Source: CAD feature listing. Evaluate the final solid. Frame: model axes, mm. Round coordinates to 2 decimals unless told otherwise and drop trailing zeros. Write each loop counter-clockwise with the first axis right and the second up, starting at its lowest first coordinate (ties: lowest second). Pieces come first, ordered by that corner, then holes.
from build123d import *

# Parameters (mm, degrees)
SKETCH1_R                = 3.175
BOSS_EXTRUDE1_DEPTH      = 69.85
BOSS_EXTRUDE1_DEPTH_BACK = 69.85


with BuildPart() as part:
    # Sketch1 → Boss-Extrude1 (new body, two sides)
    with BuildSketch(Plane.XY) as boss_extrude1_sk:
        Polygon((6.284319593, 3.777652789), (-0.129383485, 7.331206807), (-6.413703078, 3.553554018), (-6.284319593, -3.777652789), (0.129383485, -7.331206807), (6.413703078, -3.553554018), align=None)
        Circle(SKETCH1_R, mode=Mode.SUBTRACT)
    extrude(amount=BOSS_EXTRUDE1_DEPTH)
    extrude(boss_extrude1_sk.sketch, amount=-BOSS_EXTRUDE1_DEPTH_BACK)


solid = part.part
1) Section query B-B on y = 0. Return the cut outline in (x, z) (3 decimals), then the cut area to 3 significant figures.
Taken from the geometry:
outline: (-6.351, -69.85) - (-3.175, -69.85) - (-3.175, 69.85) - (-6.351, 69.85) - close; (3.175, -69.85) - (6.351, -69.85) - (6.351, 69.85) - (3.175, 69.85) - close
area: 887 mm2
2) Section query C-C on x = -4.5. Return the cut outline in (y, z), then the cut area to 3 significant figures.
Taken from the geometry:
outline: (-4.77, -69.85) - (4.7, -69.85) - (4.7, 69.85) - (-4.77, 69.85) - close
area: 1,320 mm2
3) Pull-direction query (Y, two-part tool) for faces 1 (the face through (3.228, -5.469, 0.978)), 2 (the face through (-3.228, 5.469, 0.978)), 3 (the face through (-3, -2, -69.85)), 4 (the face through (-0.69, -3.1, -0.98)); classes: released by +Y, released by -Y, zero draft, split by the parting line, or undercut.
Taken from the geometry:
face 1: released by -Y
face 2: released by +Y
face 3: zero draft
face 4: undercut
4) Section query A-A on z = 37.5. Return the cut outline in (x, y) (3 decimals), then the cut area to 3 significant figures.
Taken from the geometry:
outline: (-6.414, 3.554) - (-6.284, -3.778) - (0.129, -7.331) - (6.414, -3.554) - (6.284, 3.778) - (-0.129, 7.331) - close; hole circle Ø6.35 at (0, 0)
area: 108 mm2
5) Section query D-D on y = -6. Return the cut outline in (x, z), then the cut area to 3 significant figures.
Taken from the geometry:
outline: (-2.27, -69.85) - (2.34, -69.85) - (2.34, 69.85) - (-2.27, 69.85) - close
area: 645 mm2
6) Material intervals for line 1 (X direction, y = 3.5, z = 30.5); line 2 (Y direction, x = 0, z = -39) (3 decimals); line 3 (Y direction, x = -1.5, z = 40.5), sorted ascending.
Taken from the geometry:
line 1: x = -6.41 to 6.29
line 2: y = -7.26 to -3.175, 3.175 to 7.26
line 3: y = -6.43 to -2.8, 2.8 to 6.51
7) Contact query for flat-ended pins moving along their axis: P1, Ø3, axis at x = -3, z = 16.5, coming from the -Y side; P2, Ø3, axis at x = 3, z = -41.5, coming from the +Y side; P3, Ø2, axis at x = 3, z = -30.5, coming from the +Y side. Output: stop coordinate, or through.
Taken from the geometry:
P1: stops at y = -6.43
P2: stops at y = 6.43
P3: stops at y = 6.15
